Can you work these out from the model? Positions are in its coordinate system, mm. Face numbers are marked on the shaded views. A direction names the side the tool comes from. Coordinates: 2 decimals unless noted, no trailing zeros. Write each loop counter-clockwise with the first axis right and the second up, starting at its lowest first coordinate (ties: lowest second). Pieces come first, ordered by that corner, then holes.
Autodesk Inventor part; units mm, degrees
ref_plane "YZ Plane" through (0, 0, 0) normal (1, 0, 0) x (0, 1, 0)
ref_plane "XZ Plane" through (0, 0, 0) normal (0, 1, 0) x (-1, 0, 0)
ref_plane "XY Plane" through (0, 0, 0) normal (0, 0, 1) x (1, 0, 0)
sketch "Sketch1" plane through (0, 0, 0) normal (0, 0, 1) x (1, 0, 0)
  circle A0 centre (0, 0) radius 3.5
  line L0 (77.9423, 0) -> (38.9711, -67.5)
  line L1 (38.9711, -67.5) -> (-38.9711, -67.5)
  line L2 (-38.9711, -67.5) -> (-77.9423, 0)
  line L3 (-77.9423, 0) -> (-38.9711, 67.5)
  line L4 (-38.9711, 67.5) -> (38.9711, 67.5)
  line L5 (38.9711, 67.5) -> (77.9423, 0)
  circle A1 centre (22.5, 0) radius 2.25
  circle A2 centre (54, 0) radius 2
  circle A3 centre (15.9099, 15.9099) radius 2.25
  circle A4 centre (0, 22.5) radius 2.25
  circle A5 centre (-15.9099, 15.9099) radius 2.25
  circle A6 centre (-22.5, 0) radius 2.25
  circle A7 centre (-15.9099, -15.9099) radius 2.25
  circle A8 centre (0, -22.5) radius 2.25
  circle A9 centre (15.9099, -15.9099) radius 2.25
  circle A10 centre (46.7654, 27) radius 2
  circle A11 centre (27, 46.7654) radius 2
  circle A12 centre (0, 54) radius 2
  circle A13 centre (-27, 46.7654) radius 2
  circle A14 centre (-46.7654, 27) radius 2
  circle A15 centre (-54, 0) radius 2
  circle A16 centre (-46.7654, -27) radius 2
  circle A17 centre (-27, -46.7654) radius 2
  circle A18 centre (0, -54) radius 2
  circle A19 centre (27, -46.7654) radius 2
  circle A20 centre (46.7654, -27) radius 2
  dimension "d0" = 7
  dimension "d1" = 135
  dimension "d2" = 22.5
  dimension "d3" = 4.5
  dimension "d4" = 4
  dimension "d5" = 54
  dimension "d8" = 360
  dimension "d12" = 360
extrude "Extrusion1" add sketch "Sketch1" along normal blind 30
sketch "Sketch2" plane through (0, 0, 30) normal (0, 0, 1) x (1, 0, 0)
  circle A0 centre (0, 0) radius 3.5
  circle A1 centre (0, 0) radius 49
  dimension "d16" = 98
extrude "Extrusion2" cut sketch "Sketch2" against normal blind 15
sketch "Sketch3" plane through (0, 0, 15) normal (0, 0, 1) x (1, 0, 0)
  circle A0 centre (0, 0) radius 33
  dimension "d19" = 66
extrude "Extrusion3" cut sketch "Sketch3" against normal blind 3
sketch "Sketch4" plane through (0, 0, 12) normal (0, 0, 1) x (1, 0, 0)
  circle A0 centre (0, 0) radius 16.5
  circle A1 centre (0, 0) radius 3.5
  dimension "d22" = 33
extrude "Extrusion4" add sketch "Sketch4" along normal blind 33
sketch "Sketch5" plane through (0, 0, 45) normal (0, 0, 1) x (1, 0, 0)
  circle A0 centre (8, 0) radius 2.5
  circle A1 centre (2.4721, 7.6085) radius 2.5
  circle A2 centre (-6.4721, 4.7023) radius 2.5
  circle A3 centre (-6.4721, -4.7023) radius 2.5
  circle A4 centre (2.4721, -7.6085) radius 2.5
  point P0 (0, 0)
  dimension "d25" = 5
  dimension "d26" = 8
  dimension "d29" = 360
extrude "Extrusion5" cut sketch "Sketch5" against normal through all
sketch "Sketch6" plane through (0, 0, 0) normal (0, 0, -1) x (-1, 0, 0)
  circle A0 centre (0, 0) radius 17.5
  dimension "d33" = 35
extrude "Extrusion6" cut sketch "Sketch6" against normal blind 5
sketch "Sketch10" plane through (0, 0, 0) normal (0, 0, -1) x (-1, 0, 0)
  circle A0 centre (22.5, 0) radius 2.25
  circle A1 centre (0, 0) radius 3.5
  circle A2 centre (0, 0) radius 20.25
  circle A3 centre (0, 0) radius 24.75
  circle A4 centre (0, 0) radius 16
  circle A5 centre (0, 0) radius 29
  line L0 (29, 0) -> (16, 0)
  dimension "d38" = 13
extrude "Extrusion7" cut sketch "Sketch10" against normal blind 5 contours L0 A0 | A2 | A3 | A5 | A0 L0
sketch "Sketch11" plane through (0, 0, 12) normal (0, 0, 1) x (1, 0, 0)
  circle A0 centre (0, 0) radius 16.5
  circle A1 centre (15.9099, -15.9099) radius 2.25
  circle A2 centre (0, -22.5) radius 2.25
  circle A3 centre (-15.9099, -15.9099) radius 2.25
  circle A4 centre (-22.5, 0) radius 2.25
  circle A5 centre (-15.9099, 15.9099) radius 2.25
  circle A6 centre (0, 22.5) radius 2.25
  circle A7 centre (15.9099, 15.9099) radius 2.25
  circle A8 centre (22.5, 0) radius 2.25
  circle A9 centre (0, 0) radius 33
extrude "Extrusion8" add sketch "Sketch11" along normal up to surface (3 mm away) from surface at 0
sketch "Sketch12" plane through (0, 0, 30) normal (0, 0, 1) x (1, 0, 0)
  circle A0 centre (0, 0) radius 49
  circle A1 centre (46.7654, -27) radius 2
  circle A2 centre (27, -46.7654) radius 2
  circle A3 centre (0, -54) radius 2
  circle A4 centre (-27, -46.7654) radius 2
  circle A5 centre (-46.7654, -27) radius 2
  circle A6 centre (-54, 0) radius 2
  circle A7 centre (-46.7654, 27) radius 2
  circle A8 centre (-27, 46.7654) radius 2
  circle A9 centre (0, 54) radius 2
  circle A10 centre (27, 46.7654) radius 2
  circle A11 centre (46.7654, 27) radius 2
  circle A12 centre (54, 0) radius 2
  line L0 (38.9711, -67.5) -> (77.9423, 0)
  line L1 (77.9423, 0) -> (38.9711, 67.5)
  line L2 (38.9711, 67.5) -> (-38.9711, 67.5)
  line L3 (-38.9711, 67.5) -> (-77.9423, 0)
  line L4 (-77.9423, 0) -> (-38.9711, -67.5)
  line L5 (-38.9711, -67.5) -> (38.9711, -67.5)
extrude "Extrusion9" cut sketch "Sketch12" against normal blind 1
sketch "Sketch14" plane through (0, 0, 15) normal (0, 0, 1) x (1, 0, 0)
  circle A0 centre (0, 0) radius 3.5
  circle A1 centre (0, 0) radius 33
  circle A2 centre (15.9099, -15.9099) radius 2.25
  circle A3 centre (0, -22.5) radius 2.25
  circle A4 centre (-15.9099, -15.9099) radius 2.25
  circle A5 centre (-22.5, 0) radius 2.25
  circle A6 centre (-15.9099, 15.9099) radius 2.25
  circle A7 centre (0, 22.5) radius 2.25
  circle A8 centre (15.9099, 15.9099) radius 2.25
  circle A9 centre (22.5, 0) radius 2.25
  circle A10 centre (0, 0) radius 16.5
  circle A11 centre (0, 0) radius 49
  dimension "d45" = 66
extrude "Extrusion10" cut sketch "Sketch14" against normal blind 4 contours A11
sketch "Sketch15" plane through (0, 0, 29) normal (0, 0, 1) x (1, 0, 0)
  circle A0 centre (0, 0) radius 49 construction
  circle A1 centre (54, 0) radius 2 construction
  circle A2 centre (46.7654, 27) radius 2 construction
  circle A3 centre (27, 46.7654) radius 2 construction
  circle A4 centre (0, 54) radius 2 construction
  circle A5 centre (-27, 46.7654) radius 2 construction
  circle A6 centre (-46.7654, 27) radius 2 construction
  circle A7 centre (-54, 0) radius 2 construction
  circle A8 centre (-46.7654, -27) radius 2 construction
  circle A9 centre (-27, -46.7654) radius 2 construction
  circle A10 centre (0, -54) radius 2 construction
  circle A11 centre (27, -46.7654) radius 2 construction
  circle A12 centre (46.7654, -27) radius 2 construction
  line L0 (77.9423, 0) -> (38.9711, -67.5)
  line L1 (38.9711, 67.5) -> (77.9423, 0)
  line L2 (-38.9711, 67.5) -> (38.9711, 67.5)
  line L3 (-77.9423, 0) -> (-38.9711, 67.5)
  line L4 (-38.9711, -67.5) -> (-77.9423, 0)
  line L5 (38.9711, -67.5) -> (-38.9711, -67.5)
  line L6 (36.0844, 62.5) -> (72.1688, 0)
  line L7 (72.1688, 0) -> (36.0844, -62.5)
  line L8 (36.0844, -62.5) -> (-36.0844, -62.5)
  line L9 (-36.0844, -62.5) -> (-72.1688, 0)
  line L10 (-72.1688, 0) -> (-36.0844, 62.5)
  line L11 (-36.0844, 62.5) -> (36.0844, 62.5)
  dimension "d48" = 5
extrude "Extrusion11" add sketch "Sketch15" along normal blind 0.8
sketch "Sketch16" plane through (0, 0, 0) normal (0, 0, -1) x (-1, 0, 0)
  circle A0 centre (0, 0) radius 29
  circle A1 centre (-46.7654, -27) radius 2
  circle A2 centre (-27, -46.7654) radius 2
  circle A3 centre (0, -54) radius 2
  circle A4 centre (27, -46.7654) radius 2
  circle A5 centre (46.7654, -27) radius 2
  circle A6 centre (54, 0) radius 2
  circle A7 centre (46.7654, 27) radius 2
  circle A8 centre (27, 46.7654) radius 2
  circle A9 centre (0, 54) radius 2
  circle A10 centre (-27, 46.7654) radius 2
  circle A11 centre (-46.7654, 27) radius 2
  circle A12 centre (-54, 0) radius 2
  line L0 (-77.9423, 0) -> (-38.9711, -67.5)
  line L1 (-38.9711, -67.5) -> (38.9711, -67.5)
  line L2 (38.9711, -67.5) -> (77.9423, 0)
  line L3 (77.9423, 0) -> (38.9711, 67.5)
  line L4 (38.9711, 67.5) -> (-38.9711, 67.5)
  line L5 (-38.9711, 67.5) -> (-77.9423, 0)
  line L6 (68.1273, 0) -> (34.0637, -59)
  line L7 (34.0637, -59) -> (-34.0637, -59)
  line L8 (-34.0637, -59) -> (-68.1273, 0)
  line L9 (-68.1273, 0) -> (-34.0637, 59)
  line L10 (-34.0637, 59) -> (34.0637, 59)
  line L11 (34.0637, 59) -> (68.1273, 0)
  dimension "d51" = 118
extrude "Extrusion12" cut sketch "Sketch16" along normal through all both and the other way through all contours L5 L4 L3 L2 L1 L0
properties part number "AC05" material "ABS Plastic"
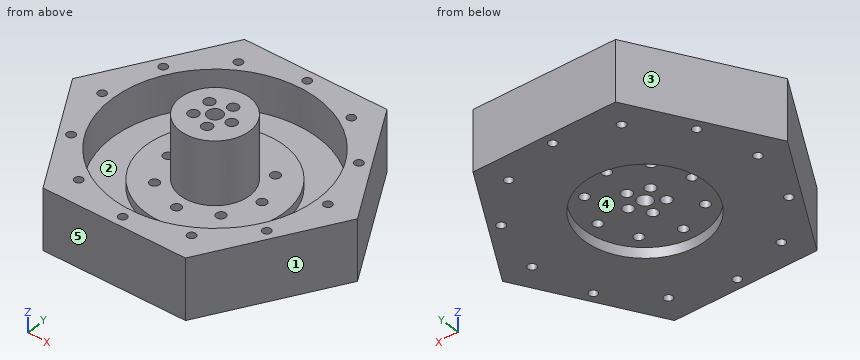
1. If we section it at B-B, the plane z = 13.5: Count the separate pieces of the cut face and the enclosed holes in it, plus the area to 3 significant figures.
2. Which directions (+Z, -Z, +X, -X, +Y, -Y) give clear straight access to the entire face, cutting with the end or side of a thin tool? Please do the marked faces 1 and 2.
3. I'm going to push flat-ended pins straight in: P1, Ø1, axis at x = -21, y = -14.5, coming from the +Z side; P2, Ø3.5, axis at x = 46.77, y = -27, coming from the -Z side; P3, Ø7, axis at x = 0, y = -22.5, coming from the -Z side; P4, Ø5, axis at x = 11.5, z = 38, coming from the +Y side. Where does each tip first touch, or does it pass through?
4. If we section it at D-D, the plane y = -27: List the corners of the cut face in (x, z) for me, plus the area to 3 significant figures.
5. If we section it at A-A, the plane y = 22.5: List the corners of the cut face in (x, z) for me, plus the area to 3 significant figures.
6. If I drill on L1, parallel to Y at x = 27, z = 8; L2, parallel to Y at x = 0, z = 1.2; L3, parallel to Y at x = 3, z = 12, over which ranges is the centre line in solid material (lowest first)?
7. We'd pull the mould along X, two halves only. Please class the marked faces 3, 4 and 5: released by +X, released by -X, zero draft, split by the parting line, or undercut.
8. If we section it at C-C, the plane x = 54: List the corners of the cut face in (y, z) for me, plus the area to 3 significant figures.
Answers:
1. separate pieces: 2
1. enclosed holes: 27
1. area: 7,520 mm2
2. face 1: +Z, -Z, +X, -Y
2. face 2: +Z
3. P1: stops at z = 15
3. P2: passes through
3. P3: stops at z = 5
3. P4: stops at y = 13.83
4. outline: (-52.54, 0) - (-48.77, 0) - (-48.77, 29) - (-52.54, 29) - close; (-44.77, 0) - (-10.58, 0) - (-10.58, 5) - (10.58, 5) - (10.58, 0) - (44.77, 0) - (44.77, 29) - (40.89, 29) - (40.89, 11) - (18.97, 11) - (18.97, 15) - (-18.97, 15) - (-18.97, 11) - (-40.89, 11) - (-40.89, 29) - (-44.77, 29) - close; (48.77, 0) - (52.54, 0) - (52.54, 29) - (48.77, 29) - close
4. area: 1,390 mm2
5. outline: (-55.14, 0) - (-18.3, 0) - (-18.3, 5) - (-2.25, 5) - (-2.25, 15) - (-24.14, 15) - (-24.14, 11) - (-43.53, 11) - (-43.53, 29) - (-55.14, 29) - close; (2.25, 5) - (18.3, 5) - (18.3, 0) - (55.14, 0) - (55.14, 29) - (43.53, 29) - (43.53, 11) - (24.14, 11) - (24.14, 15) - (2.25, 15) - close
5. area: 1,600 mm2
6. L1: y = -59 to -48.77, -44.77 to 44.77, 48.77 to 59
6. L2: y = -59 to -56, -52 to -29, 29 to 52, 56 to 59
6. L3: y = -59 to -48.91, -32.86 to -10.05, -5.16 to -1.8, 1.8 to 5.16, 10.05 to 32.86, 48.91 to 59
7. face 3: released by -X
7. face 4: undercut
7. face 5: zero draft
8. outline: (-24.47, 0) - (-2, 0) - (-2, 29) - (-24.47, 29) - close; (2, 0) - (24.47, 0) - (24.47, 29) - (2, 29) - close
8. area: 1,300 mm2
